Geometry check sheet. Reference: the model listing, model coordinates, mm. A direction names the side the tool comes from. Round coordinates to 2 decimals unless told otherwise and drop trailing zeros. Write each loop counter-clockwise with the first axis right and the second up, starting at its lowest first coordinate (ties: lowest second). Pieces come first, ordered by that corner, then holes. Notation, with made-up numbers: (-23.75, 45) -> (34.25, 45) arc R21 ccw to (34.25, 58) -> close; hole circle Ø2 at (11.25, -31). An arc over 180 degrees is marked (long way). Use a Markdown table: item, result.
```python
from build123d import *

# Parameters (mm, degrees)
F0_W     = 495.3
F0_H     = 488.95
F1_DEPTH = 107.95
F2_W     = 254
F2_H     = 387.35
F3_DEPTH = 6.35
F4_W     = 50.8
F4_H     = 19.05
F4_H_2   = 18.415
F5_DEPTH = 25.4
F6_W     = 106.6431775689
F6_H     = 105.2582077682
F6_W_2   = 47.7816872299
F6_H_2   = 191.8192440644
F7_DEPTH = 12.7


with BuildPart() as f1:
    # F0 (on Front) → F1 (new body, symmetric)
    with BuildSketch(Plane.XZ):
        Rectangle(F0_W, F0_H)
    extrude(amount=F1_DEPTH, both=True)

    # F2 (on face) → F3 (cut)
    with BuildSketch(Plane.XZ.offset(107.95)):
        with Locations((-76.2, -12.7)):
            Rectangle(F2_W, F2_H)
    extrude(amount=-F3_DEPTH, mode=Mode.SUBTRACT)

    # F4 (on face) → F5 (join)
    with BuildSketch(Plane(origin=(0, 0, -244.475), x_dir=(1, 0, 0), z_dir=(0, 0, -1))):
        with Locations((-203.2, 95.885)):
            Rectangle(F4_W, F4_H)
        with Locations((177.8, 95.885)):
            Rectangle(F4_W, F4_H)
        with Locations((177.8, -96.2025)):
            Rectangle(F4_W, F4_H_2)
        with Locations((-203.2, -95.885)):
            Rectangle(F4_W, F4_H)
    extrude(amount=F5_DEPTH)

    # F6 (on face) → F7 (cut)
    with BuildSketch(Plane(origin=(-247.65, 0, 0), x_dir=(0, -1, 0), z_dir=(-1, 0, 0))):
        with Locations((-1.0387524962, -84.1373149306)):
            Rectangle(F6_W, F6_H)
        with Locations((-58.1690315157, 105.9507015161)):
            Rectangle(F6_W_2, F6_H_2)
    extrude(amount=-F7_DEPTH, mode=Mode.SUBTRACT)


solid = f1.part
```
(1) Gauge pin test, flat ends, axial feed: pin 1 Ø7.5 at (x, z) = (-214.5, -253.5) entering from +Y; pin 2 Ø5.5 at (y, z) = (-98.5, -258) entering from +X; pin 3 Ø2 at (x, y) = (-197.5, 39) entering from -Z (3 decimals). Record the tip position at first contact, or that the pin passes through.
A:
| item | result |
|---|---|
| pin 1 | stops at y = 105.41 |
| pin 2 | stops at x = 203.2 |
| pin 3 | stops at z = -244.475 |
(2) Section check B-B on x = -210.5. Record the cut outline in (y, z) (3 decimals), plus the area to 3 significant figures.
A:
| item | result |
|---|---|
| outline | (-107.95, -244.475) -> (-105.41, -244.475) -> (-105.41, -269.875) -> (-86.36, -269.875) -> (-86.36, -244.475) -> (86.36, -244.475) -> (86.36, -269.875) -> (105.41, -269.875) -> (105.41, -244.475) -> (107.95, -244.475) -> (107.95, 244.475) -> (-107.95, 244.475) -> close |
| area | 107,000 mm2 |
(3) Access from +Z, -Z, +X, -X, +Y, -Y to the whole of each face (thin tool, end or side, straight path). Record for faces 1 (the face through (203.2, 96, -257)), 2 (the face through (-204, -86.36, -257)), 3 (the face through (-241, -52.283, -85)), 4 (the face through (-228.6, -96, -257)).
A:
| item | result |
|---|---|
| face 1 | -Z, +X, +Y, -Y |
| face 2 | -Z, +X, -X |
| face 3 | -X |
| face 4 | -Z, -X, +Y, -Y |
(4) Release check for a two-part mould opening along Y. For faces 5 (the face through (177, 105.41, -257)), 6 (the face through (177, -105.41, -257)), 7 (the face through (-241, 59, 10.041)), 8 (the face through (247.65, -2, -3)) record: +Y half, -Y half, draft (parallel to the pull), parting line (faces both ways), or undercut.
A:
| item | result |
|---|---|
| face 5 | +Y half |
| face 6 | -Y half |
| face 7 | undercut |
| face 8 | draft |
(5) Section check C-C on y = -15. Record the cut outline in (x, z) (3 decimals), plus the area to 3 significant figures.
A:
| item | result |
|---|---|
| outline | (-247.65, -244.475) -> (247.65, -244.475) -> (247.65, 244.475) -> (-247.65, 244.475) -> (-247.65, -31.508) -> (-234.95, -31.508) -> (-234.95, -136.766) -> (-247.65, -136.766) -> close |
| area | 241,000 mm2 |
(6) Section check A-A on z = 4. Record the cut outline in (x, y), plus the area to 3 significant figures.
A:
| item | result |
|---|---|
| outline | (-247.65, -107.95) -> (-203.2, -107.95) -> (-203.2, -101.6) -> (50.8, -101.6) -> (50.8, -107.95) -> (247.65, -107.95) -> (247.65, 107.95) -> (-247.65, 107.95) -> close |
| area | 105,000 mm2 |
(7) Section check D-D on y = -93. Record the cut outline in (x, z) (3 decimals), plus the area to 3 significant figures.
A:
| item | result |
|---|---|
| outline | (-247.65, -244.475) -> (-228.6, -244.475) -> (-228.6, -269.875) -> (-177.8, -269.875) -> (-177.8, -244.475) -> (152.4, -244.475) -> (152.4, -269.875) -> (203.2, -269.875) -> (203.2, -244.475) -> (247.65, -244.475) -> (247.65, 244.475) -> (-247.65, 244.475) -> close |
| area | 245,000 mm2 |
(8) Thickness scan on line 1 (Z direction, x = -69.5, y = -9) (3 decimals); line 2 (X direction, y = 75, z = 192.5); line 3 (Y direction, x = -131, z = 119.5). Record the ranges inside material, lowest first.
A:
| item | result |
|---|---|
| line 1 | z = -244.475 to 244.475 |
| line 2 | x = -234.95 to 247.65 |
| line 3 | y = -101.6 to 107.95 |
